Geometry: final body of the model. Coordinates: model frame, mm. A direction names the side the tool comes from. Give positions to 0.01 mm unless a question says otherwise; leave off trailing zeros. Loops run counter-clockwise (first coordinate to the right, second up) from the corner with the lowest first, then second, coordinate; pieces in that order, holes last.
Autodesk Fusion 360 part; units mm, degrees
sketch "Sketch1" plane through (0, 0, 0) normal (0, 0, 1) x (1, 0, 0)
  line L0 (60, -60) -> (-60, -60)
  line L1 (-60, -60) -> (-60, 60)
  line L2 (-60, 60) -> (60, 60)
  line L3 (60, 60) -> (60, -60)
  line L4 (60, -60) -> (-60, 60) construction
  line L5 (-60, -60) -> (60, 60) construction
  line L6 (25, 20) -> (-25, 20)
  line L7 (-25, 20) -> (-25, -20)
  line L8 (-25, -20) -> (25, -20)
  line L9 (25, -20) -> (25, 20)
  line L10 (25, 20) -> (-25, -20) construction
  line L11 (-25, 20) -> (25, -20) construction
  line L12 (60, 5) -> (-50, 60)
  line L13 (60, -5) -> (-50, -60)
  line L14 (-60, 50) -> (-25, 5)
  line L15 (-60, -50) -> (-25, -5)
  dimension "d1" = 120
  dimension "d2" = 120
  dimension "d6" = 50
  dimension "d7" = 40
  dimension "d29" = 5
  dimension "d30" = 5
  dimension "d31" = 10
  dimension "d34" = 10
  dimension "d41" = 10
  dimension "d42" = 10
extrude "Extrude1" add sketch "Sketch1" along normal blind 3 contours L0 L1 L2 L3 L6 L7 L8 L9 L12 L13 L14 L15 | L6 L7 L8 L9
sketch "Sketch2" plane through (0, 0, 3) normal (0, 0, 1) x (-1, 0, 0)
  line L0 (60, 50) -> (60, 60)
  line L1 (60, 60) -> (50, 60)
  line L2 (50, 60) -> (-60, 5)
  line L3 (-60, 5) -> (-60, -5)
  line L4 (-60, -5) -> (50, -60)
  line L5 (50, -60) -> (60, -60)
  line L6 (60, -60) -> (60, -50)
  line L7 (25, 5) -> (60, 50)
  line L8 (60, -50) -> (25, -5)
  line L9 (25, -5) -> (25, 5)
  point P0 (-7.5, -8)
  point P1 (19, -10)
  point P2 (7.5, -8)
  point P3 (-7.5, 8)
  point P4 (7.5, 8)
  point P5 (-19, -10)
  point P6 (19, 10)
  point P7 (-19, 10)
  point P8 (55, -55)
  point P9 (-55, 0)
  point P10 (55, 55)
  dimension "d12" = 7.5
  dimension "d13" = 8
  dimension "d14" = 19
  dimension "d15" = 10
  dimension "d18" = 15
  dimension "d19" = 16
  dimension "d22" = -38
  dimension "d23" = 20
  dimension "d47" = 5
  dimension "d48" = 5
  dimension "d49" = 5
  dimension "d50" = 5
  dimension "d51" = 5
hole "Hole1" at (-19, 10, 3) at (-7.5, 8, 3) at (7.5, 8, 3) at (19, 10, 3) at (19, -10, 3) at (7.5, -8, 3) at (-7.5, -8, 3) at (-19, -10, 3) at (-55, -55, 3) at (55, 0, 3) at (-55, 55, 3) direction (0, 0, -1) diameter 3.2 depth 30 tip angle 118
Item 1: Section query B-B on x = 55. Return loops of the section in (y, z).
Values follow:
outline: (-7.5, 0) - (-1.6, 0) - (-1.6, 3) - (-7.5, 3) - close; (1.6, 0) - (7.5, 0) - (7.5, 3) - (1.6, 3) - close
Item 2: Section query A-A on y = 0. Return loops of the section in (x, z).
Values follow:
outline: (-25, 0) - (53.4, 0) - (53.4, 3) - (-25, 3) - close; (56.6, 0) - (60, 0) - (60, 3) - (56.6, 3) - close
Item 3: Ray query, probe 1 along X at (y, z) = (10, 1.1); probe 2 along X at (y, z) = (0, 1.35); probe 3 along Y at (x, z) = (-55, 1.1). Return the intervals inside material, ascending.
Values follow:
probe 1: x = -28.89 to -20.6, -17.4 to 17.4, 20.6 to 50
probe 2: x = -25 to 53.4, 56.6 to 60
probe 3: y = -60 to -56.6, -53.4 to -43.57, 43.57 to 53.4, 56.6 to 60
Item 4: Draft query along Y for faces 3 (the face through (-60, 55, 1)), 4 (the face through (6, -32, 1)), 5 (the face through (9.06, -7.65, 1.48)), 6 (the face through (6, 32, 1)). Return one class per face: +Y half, -Y half, draft (parallel to the pull), parting line (faces both ways), or undercut.
Values follow:
face 3: draft
face 4: -Y half
face 5: undercut
face 6: +Y half
Item 5: Section query D-D on x = -19. Return loops of the section in (y, z).
Values follow:
outline: (-44.5, 0) - (-11.6, 0) - (-11.6, 3) - (-44.5, 3) - close; (-8.4, 0) - (8.4, 0) - (8.4, 3) - (-8.4, 3) - close; (11.6, 0) - (44.5, 0) - (44.5, 3) - (11.6, 3) - close
Item 6: Section query C-C on z = 1.2. Give the number of separate pieces and of enclosed holes in the cut face, plus the area to 3 significant figures.
Values follow:
separate pieces: 1
enclosed holes: 11
area: 6,340 mm2
Item 7: Set-up query: faces 1 (the face through (-20.586, 10.208, 1.479)), 2 (the face through (-42.745, 27.815, 1.479)). Return all of +Z, -Z, +X, -X, +Y, -Y with unobstructed straight access to the full face (end or side cutting, diameter ignored); none if empty.
Values follow:
face 1: +Z, -Z
face 2: +Z, -Z, -X
